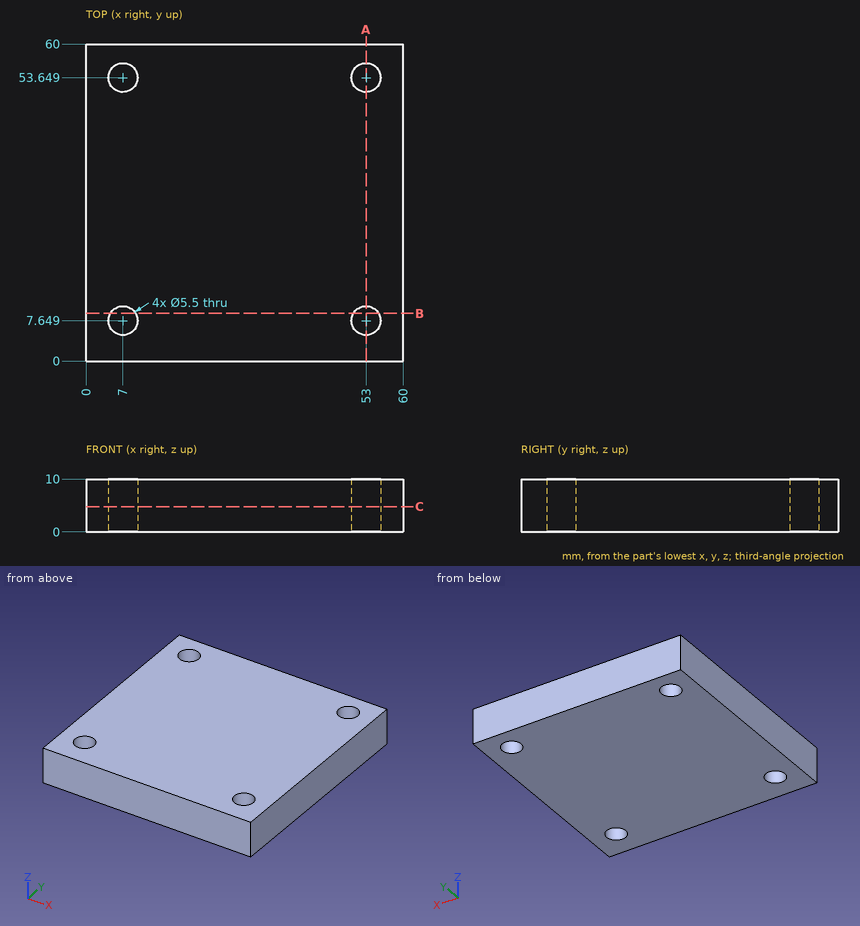
Check sheet for the drawn part. Datum: minimum x, y, z corner. Units: mm. Give positions to 0.01 mm unless a question says otherwise; leave off trailing zeros. Write each loop counter-clockwise with the first axis right and the second up, starting at its lowest first coordinate (ties: lowest second). Pieces come first, ordered by that corner, then holes.
(1) Material ranges on line 1 (Y direction, x = 7, z = 3.75); line 2 (X direction, y = 8.5, z = 5.5) (1 decimal), recorded low to high.
(2) Cross-section at A-A (x = 53). Enter the section's corners in (y, z).
(3) Cross-section at C-C (z = 4.75). Enter the section's corners in (x, y).
(4) Cross-section at B-B (y = 9). Enter the section's corners in (x, z) (1 decimal).
(5) Gauge pin test, flat end, axial feed: pin 1 (4.5 mm diameter, centred on x = 7, y = 53.65, fed in from +Z). Record the tip position at first contact, or that the pin passes through.
Worked out:
1. line 1: y = 0 to 4.9, 10.4 to 50.9, 56.4 to 60
1. line 2: x = 0 to 4.4, 9.6 to 50.4, 55.6 to 60
2. outline: (0, 0) - (4.9, 0) - (4.9, 10) - (0, 10) - close; (10.4, 0) - (50.9, 0) - (50.9, 10) - (10.4, 10) - close; (56.4, 0) - (60, 0) - (60, 10) - (56.4, 10) - close
3. outline: (0, 0) - (60, 0) - (60, 60) - (0, 60) - close; hole circle Ø5.5 at (7, 7.65); hole circle Ø5.5 at (7, 53.65); hole circle Ø5.5 at (53, 7.65); hole circle Ø5.5 at (53, 53.65)
4. outline: (0, 0) - (4.6, 0) - (4.6, 10) - (0, 10) - close; (9.4, 0) - (50.6, 0) - (50.6, 10) - (9.4, 10) - close; (55.4, 0) - (60, 0) - (60, 10) - (55.4, 10) - close
5. pin 1: passes through
